Part model, mm, in its own coordinate system. Give positions to 0.01 mm unless a question says otherwise; leave off trailing zeros. Order: outer loops, then holes, each group sorted by start corner. A loop starts at its lowest first (then second) coordinate and runs counter-clockwise, first axis right, second up. Notation, with made-up numbers: (-0.75, 19) -> (43.25, 19) arc R31 cw to (43.25, 45) -> close; hole circle Ø4 at (-39.5, 15). An arc over 180 degrees is marked (long way). Write item = value, one per line. Start each with the question number.
Item 1: Pull direction Y, two halves, no side cores. Call faces 1 (the face through (2.15, -3.373, -32.197)), 2 (the face through (2.195, 0.706, -65.288)): +Y half, -Y half, draft (parallel to the pull), parting line (faces both ways), or undercut.
Item 2: Band-saw the part on A-A on z = -8.5. Write the cut outline in (x, y), plus the area to 3 significant figures.
Item 3: Drill centre lines: line 1 along Y through (x, z) = (0, -22); line 2 along Y through (x, z) = (-2.75, -39). Where is each one in solid material? Low to high.
Item 4: Flat gauge pins, fed straight in: P1, Ø1.5, axis at x = -1.5, z = -27, coming from the +Y side; P2, Ø4, axis at y = 3, z = -27, coming from the -X side; P3, Ø1.5, axis at x = 2.5, z = -22, coming from the -Y side. Where does each tip first touch, or does it go through?
```python
from build123d import *

# Parameters (mm, degrees)
F4_SIZE  = 0.3
F6_START = -30
F5_R     = 3.25
F6_DEPTH = 7.1198021535


with BuildPart() as f3:
    # F2 (on Front) → F3 (revolve)
    with BuildSketch(Plane.XZ):
        Polygon((4, 0), (3.2, 0), (3.2, -64.5381197846), (0, -66.3856406461), (0, -67.3094010768), (4, -65), align=None)
    revolve(axis=Axis((0, 0, -32.7149666846), (0, 0, -1)))

    # F4
    f4_edges = [f3.edges().sort_by_distance(p)[0] for p in [
        (-4, 0, 0),
        (-3.2, 0, 0),
    ]]
    chamfer(f4_edges, length=F4_SIZE)

    # F5 (on line) → F6 (cut)
    with BuildSketch(Plane(origin=(0, 0, 0), x_dir=(1, 0, 0), z_dir=(0, -0.8660254038, 0.5)).offset(F6_START)):
        with Locations((0, -53.791651246)):
            Circle(F5_R)
    extrude(amount=-F6_DEPTH, mode=Mode.SUBTRACT)


solid = f3.part
```
Values found:
q1.face_1 = parting line
q1.face_2 = undercut
q2.outline = circle Ø8 at (0, 0); hole circle Ø6.4 at (0, 0)
q2.area = 18.1 mm^2
q3.line_1 = -4 to -3.2, 3.2 to 4
q3.line_2 = -2.9 to -1.64, 1.64 to 2.9
q4.P1 = 3.93
q4.P2 = -3.87
q4.P3 = -3.6
